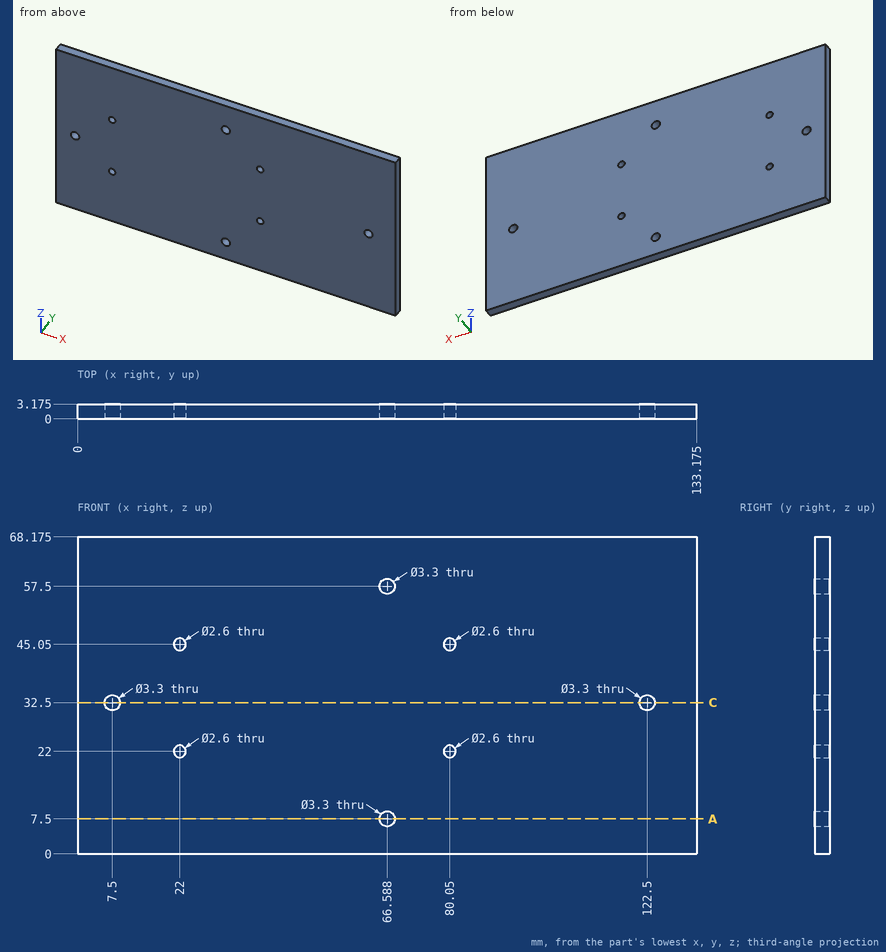
Check sheet for the drawn part. Datum: minimum x, y, z corner. Units: mm. Round coordinates to 2 decimals unless told otherwise and drop trailing zeros. Write each loop counter-clockwise with the first axis right and the second up, starting at its lowest first coordinate (ties: lowest second). Pieces come first, ordered by that corner, then holes. Notation, with made-up numbers: (-6.75, 53.5) - (43.25, 53.5) arc R19 ccw to (43.25, 61.5) - close; hole circle Ø7 at (-12.5, -16). An arc over 180 degrees is marked (long way). Return JSON: item names as keys, results as strings.
Q1. Cross-section at A-A (z = 7.5). Record the boundary of the cut face in (x, y) (1 decimal).
Returned:
{"outline": "(0, 0) - (64.9, 0) - (64.9, 3.2) - (0, 3.2) - close; (68.2, 0) - (133.2, 0) - (133.2, 3.2) - (68.2, 3.2) - close"}
Q2. Depth check by flat-ended pin: P1, Ø2, axis at x = 80.05, z = 22, coming from the +Y side. Enter the tip coordinate at first touch or a pass-through.
Returned:
{"P1": "passes through"}
Q3. Cross-section at C-C (z = 32.5). Give the number of separate pieces and of enclosed holes in the cut face, then the cut area to 3 significant figures.
Returned:
{"separate pieces": "3", "enclosed holes": "0", "area": "402 mm²"}
